Input: part model. Units: mm. Frame: model coordinates. A direction names the side the tool comes from. Give positions to 0.01 mm unless a question says otherwise; leave off trailing zeros. Write each loop counter-clockwise with the first axis right and the second up, starting at its lowest first coordinate (ties: lowest second). Pieces come first, ordered by that corner, then holes.
```python
from build123d import *

# Parameters (mm, degrees)
SKETCH_W                = 57
SKETCH_H                = 27
PAD_DEPTH               = 2
PAD001_DEPTH            = 3
PAD001_MIRRORED_2_DEPTH = 3
POCKET_DEPTH            = 2
SKETCH003_W             = 57
SKETCH003_H             = 27
SKETCH003_W_2           = 55
SKETCH003_H_2           = 25
PAD002_DEPTH            = 4
SKETCH004_W             = 1
SKETCH004_H             = 8.5
POCKET001_DEPTH         = 3.7
SKETCH005_W             = 57
SKETCH005_H             = 27
PAD003_DEPTH            = 2
SKETCH006_W             = 3
SKETCH006_H             = 21
POCKET002_DEPTH         = 2
LINEARPATTERN_COUNT     = 10
LINEARPATTERN_PITCH     = 6
SKETCH007_R             = 4
PAD004_DEPTH            = 12
SKETCH008_R             = 3.25
POCKET003_DEPTH         = 12


with BuildPart() as part:
    # Sketch → Pad (new body)
    with BuildSketch(Plane.XY):
        Rectangle(SKETCH_W, SKETCH_H)
    extrude(amount=PAD_DEPTH)

    # Sketch001 (on Face6 of Pad) → Pad001 (join)
    with BuildSketch(Plane.XY.offset(2)):
        Polygon((-26.5, 11.5), (-23.5, 11.5), (-23.5, 10.5), (-25.7, 10.5), (-25.7, 8.5), (-26.5, 8.5), align=None)
    pad001 = extrude(amount=PAD001_DEPTH)

    # Sketch001 Mirrored 2 → Pad001 Mirrored 2 (add)
    with BuildSketch(Plane(origin=(0, 0, 2), x_dir=(-1, 0, 0), z_dir=(0, 0, -1))):
        Polygon((-26.5, 11.5), (-23.5, 11.5), (-23.5, 10.5), (-25.7, 10.5), (-25.7, 8.5), (-26.5, 8.5), align=None)
    pad001_mirrored_2 = extrude(amount=-PAD001_MIRRORED_2_DEPTH)

    # Mirrored001: Pad001, Pad001 Mirrored 2 across Sketch001 H_Axis
    add(pad001.mirror(Plane(origin=(0, 0, 2), x_dir=(0, 0, 1), z_dir=(0, 1, 0))))
    add(pad001_mirrored_2.mirror(Plane(origin=(0, 0, 2), x_dir=(0, 0, 1), z_dir=(0, 1, 0))))

    # Sketch002 (on Face5 of MultiTransform) → Pocket (cut)
    with BuildSketch(Plane.XY.offset(2)):
        Polygon((23.5, 10.5), (25.5, 8.5), (25.5, -8.5), (23.5, -10.5), (-23.5, -10.5), (-25.5, -8.5), (-25.5, 8.5), (-23.5, 10.5), align=None)
    extrude(amount=-POCKET_DEPTH, mode=Mode.SUBTRACT)

    # Sketch003 (on Face5 of Pocket) → Pad002 (join)
    with BuildSketch(Plane.XY.offset(2)):
        Rectangle(SKETCH003_W, SKETCH003_H)
        Rectangle(SKETCH003_W_2, SKETCH003_H_2, mode=Mode.SUBTRACT)
    extrude(amount=PAD002_DEPTH)

    # Sketch004 (on Face17 of Pad002) → Pocket001 (cut)
    with BuildSketch(Plane.XY.offset(6)):
        with Locations((-28, 0)):
            Rectangle(SKETCH004_W, SKETCH004_H)
    extrude(amount=-POCKET001_DEPTH, mode=Mode.SUBTRACT)

    # Sketch005 (on Face4 of Pocket001) → Pad003 (join)
    with BuildSketch(Plane(origin=(0, 0, 0), x_dir=(1, 0, 0), z_dir=(0, 0, -1))):
        Rectangle(SKETCH005_W, SKETCH005_H)
    extrude(amount=PAD003_DEPTH)

    # Sketch006 (on Face11 of Pad003) → Pocket002 (cut)
    with BuildSketch(Plane(origin=(0, 0, -2), x_dir=(1, 0, 0), z_dir=(0, 0, -1))):
        with Locations((-24, 0)):
            Rectangle(SKETCH006_W, SKETCH006_H)
    pocket002 = extrude(amount=-POCKET002_DEPTH, mode=Mode.SUBTRACT)

    # LinearPattern: Pocket002 ×10
    with Locations(*[(i * LINEARPATTERN_PITCH, 0, 0) for i in range(1, LINEARPATTERN_COUNT)]):
        add(pocket002, mode=Mode.SUBTRACT)

    # Sketch007 (on Face62 of LinearPattern) → Pad004 (join)
    with BuildSketch(Plane(origin=(0, 0, 0), x_dir=(1, 0, 0), z_dir=(0, 0, -1))):
        with Locations((-12, 0)):
            Circle(SKETCH007_R)
    pad004 = extrude(amount=PAD004_DEPTH)

    # Sketch008 (on Face72 of Pad004) → Pocket003 (cut)
    with BuildSketch(Plane(origin=(0, 0, -12), x_dir=(1, 0, 0), z_dir=(0, 0, -1))):
        with Locations((-12, 0)):
            Circle(SKETCH008_R)
    pocket003 = extrude(amount=-POCKET003_DEPTH, mode=Mode.SUBTRACT)

    # Mirrored002: Pad004 across Sketch007 V_Axis
    add(pad004.mirror(Plane(origin=(0, 0, 0), x_dir=(0, 0, -1), z_dir=(1, 0, 0))))

    # Mirrored003: Pocket003 across Sketch008 V_Axis
    add(pocket003.mirror(Plane(origin=(0, 0, -12), x_dir=(0, 0, -1), z_dir=(1, 0, 0))), mode=Mode.SUBTRACT)


solid = part.part
```
Q1. Material intervals for line 1 along X through (y, z) = (0, -3); line 2 along Y through (x, z) = (-12, -4.75); line 3 along Y through (x, z) = (-3, 3.5), sorted ascending.
Q2. Section D-D, the plane y = 0. Give the number of separate pieces and of enclosed holes in the cut face, then the cut area to 3 significant figures.
Q3. Section C-C, the plane z = -2.75. Return the cut outline in (x, y).
Q4. Mould query, pull axis X, two halves, no side actions, for faces 1 (the flat face through (-28, -4.25, 4)), 2 (the flat face through (10.5, -7, -1)). Classes: +X half, -X half, draft (parallel to the pull), parting line (faces both ways), or undercut.
Q5. Section B-B, the plane x = -12. Return the cut outline in (y, z), then the cut area to 3 significant figures.
Q6. Section A-A, the plane x = -5.5. Return the cut outline in (y, z).
Q7. Access query for faces 3 (the flat face through (-1.5, 0, -1)), 4 (the flat face through (25.5, 0, 0)), 5 (the flat face through (-26.5, 10, 3)). Directions: +Z, -Z, +X, -X, +Y, -Y. A direction counts if a zero-diameter tool reaches every point of the face in a straight line with its end or side. Return the directions, or none.
Q8. Pin query (flat end, axial travel): pin 1 (1.6 mm diameter, centred on x = -25, y = 9.5, fed in from -Z); pin 2 (3 mm diameter, centred on x = -8, y = 7.5, fed in from +Z); pin 3 (5 mm diameter, centred on x = -3.5, z = -3.5, fed in from -Y); pin 4 (0.9 mm diameter, centred on x = -24.5, y = 9.5, fed in from +Z). Return the tip coordinate at first contact, or that it passes through.
Solutions:
1. line 1: x = -16 to -15.25, -8.75 to -8, 8 to 8.75, 15.25 to 16
1. line 2: y = -4 to -3.25, 3.25 to 4
1. line 3: y = -13.5 to -12.5, 12.5 to 13.5
2. separate pieces: 10
2. enclosed holes: 0
2. area: 92.3 mm2
3. outline: circle Ø8 at (-12, 0); circle Ø8 at (12, 0); hole circle Ø6.5 at (-12, 0); hole circle Ø6.5 at (12, 0)
4. face 1: draft
4. face 2: undercut
5. outline: (-13.5, -2) - (-10.5, -2) - (-10.5, 2) - (-12.5, 2) - (-12.5, 6) - (-13.5, 6) - close; (-4, -12) - (-3.25, -12) - (-3.25, 0) - (-4, 0) - close; (3.25, -12) - (4, -12) - (4, 0) - (3.25, 0) - close; (10.5, -2) - (13.5, -2) - (13.5, 6) - (12.5, 6) - (12.5, 2) - (10.5, 2) - close
5. area: 50.0 mm2
6. outline: (-13.5, -2) - (-10.5, -2) - (-10.5, 2) - (-12.5, 2) - (-12.5, 6) - (-13.5, 6) - close; (10.5, -2) - (13.5, -2) - (13.5, 6) - (12.5, 6) - (12.5, 2) - (10.5, 2) - close
7. face 3: +Z, -Z
7. face 4: -Z
7. face 5: +Z
8. pin 1: stops at z = -2
8. pin 2: stops at z = 0
8. pin 3: stops at y = -13.5
8. pin 4: stops at z = 2
